The listing builds one solid part. Answer for the finished solid, in the listing's coordinates (mm). A direction names the side the tool comes from. Coordinates: 2 decimals unless noted, no trailing zeros. Order: outer loops, then holes, each group sorted by start corner. A loop starts at its lowest first (then second) coordinate and runs counter-clockwise, first axis right, second up. Notation, with made-up numbers: (61.25, 38) - (102.25, 38) arc R23 cw to (102.25, 60) - close; hole circle Ø5 at (-6.5, -14.5). An arc over 180 degrees is marked (long way). Use a Markdown table: item, result. Add a question column.
Item 1: Find the intervals of material crossed by line 1 along Z through (x, y) = (-6.5, 19); line 2 along X through (y, z) = (19, -5.5); line 3 along Z through (x, y) = (3, 23), in increasing order.
Item 2: For faces 1 (the flat face through (-28, 15, 0)), 2 (the flat face through (0, 26, -21)), 3 (the flat face through (16, 11, 0)), determine the directions among +Z, -Z, +X, -X, +Y, -Y from which every point of the face is accessible in a straight line to the end or side of a thin tool.
Item 3: The mould has two halves that part along Z. Classify faces 4 (the flat face through (0, 15, -25)), 5 (the flat face through (28, 15, 0)), 6 (the flat face through (0, 11, -13)): released by +Z, released by -Z, zero draft, split by the parting line, or undercut.
Item 4: A flat-ended cylindrical pin translates along its axis: P1, Ø8, axis at x = -17.5, z = 0, coming from the +Y side. Find the tip coordinate at first contact, or state that the pin passes through.
Item 5: The part is cut by section A-A, the plane x = 10. Give the vertices of the cut face in (y, z), then the cut area to 3 significant figures.
Item 6: The part is cut by section B-B, the plane z = -10.5. Give the vertices of the cut face in (x, y), then the cut area to 3 significant figures.
Item 7: The part is cut by section D-D, the plane x = 22. Give the vertices of the cut face in (y, z).
Item 8: The part is cut by section C-C, the plane y = 24. Give the vertices of the cut face in (x, z).
from build123d import *

# Parameters (mm, degrees)
SKETCH1_W               = 56
SKETCH1_H               = 50
BOSS_EXTRUDE1_DEPTH     = 30
SKETCH3_W               = 48
SKETCH3_H               = 42
CUT_EXTRUDE1_DEPTH      = 8
CUT_EXTRUDE2_DEPTH      = 44.508619836
CUT_EXTRUDE2_DEPTH_BACK = 44.508619836
SKETCH5_W               = 32
SKETCH5_H               = 26


with BuildPart() as part:
    # Sketch1 → Boss-Extrude1 (new body)
    with BuildSketch(Plane(origin=(0, 0, 0), x_dir=(1, 0, 0), z_dir=(0, 1, 0))):
        Rectangle(SKETCH1_W, SKETCH1_H)
    extrude(amount=BOSS_EXTRUDE1_DEPTH)

    # Sketch3 → Cut-Extrude1 (cut)
    with BuildSketch(Plane(origin=(0, 30, 0), x_dir=(1, 0, 0), z_dir=(0, 1, 0))):
        Rectangle(SKETCH3_W, SKETCH3_H)
    extrude(amount=-CUT_EXTRUDE1_DEPTH, mode=Mode.SUBTRACT)

    # Sketch5 → Cut-Extrude2 (cut, two sides: drawn at the far end of the back side and taken through both)
    with BuildSketch(Plane(origin=(0, 22, 0), x_dir=(1, 0, 0), z_dir=(0, 1, 0)).offset(-CUT_EXTRUDE2_DEPTH_BACK)):
        Rectangle(SKETCH5_W, SKETCH5_H)
    extrude(amount=CUT_EXTRUDE2_DEPTH + CUT_EXTRUDE2_DEPTH_BACK, mode=Mode.SUBTRACT)


solid = part.part
Solution:
| question | item | result |
|---|---|---|
| 1 | line 1 | z = -25 to -13, 13 to 25 |
| 1 | line 2 | x = -28 to -16, 16 to 28 |
| 1 | line 3 | z = -25 to -21, 21 to 25 |
| 2 | face 1 | +Z, -Z, -X, +Y, -Y |
| 2 | face 2 | +Y |
| 2 | face 3 | +Y, -Y |
| 3 | face 4 | released by -Z |
| 3 | face 5 | zero draft |
| 3 | face 6 | undercut |
| 4 | P1 | stops at y = 22 |
| 5 | outline | (0, -25) - (30, -25) - (30, -21) - (22, -21) - (22, -13) - (0, -13) - close; (0, 13) - (22, 13) - (22, 21) - (30, 21) - (30, 25) - (0, 25) - close |
| 5 | area | 592 mm2 |
| 6 | outline | (-28, 0) - (-16, 0) - (-16, 22) - (-24, 22) - (-24, 30) - (-28, 30) - close; (16, 0) - (28, 0) - (28, 30) - (24, 30) - (24, 22) - (16, 22) - close |
| 6 | area | 592 mm2 |
| 7 | outline | (0, -25) - (30, -25) - (30, -21) - (22, -21) - (22, 21) - (30, 21) - (30, 25) - (0, 25) - close |
| 8 | outline | (-28, -25) - (28, -25) - (28, 25) - (-28, 25) - close; hole (-24, -21) - (24, -21) - (24, 21) - (-24, 21) - close |
